Geometry: final body of the model. Coordinates: model frame, mm. Face numbers are marked on the shaded views. Coordinates: 2 decimals unless noted, no trailing zeros. Write each loop counter-clockwise with the first axis right and the second up, starting at its lowest first coordinate (ties: lowest second). Pieces come first, ordered by that corner, then holes.
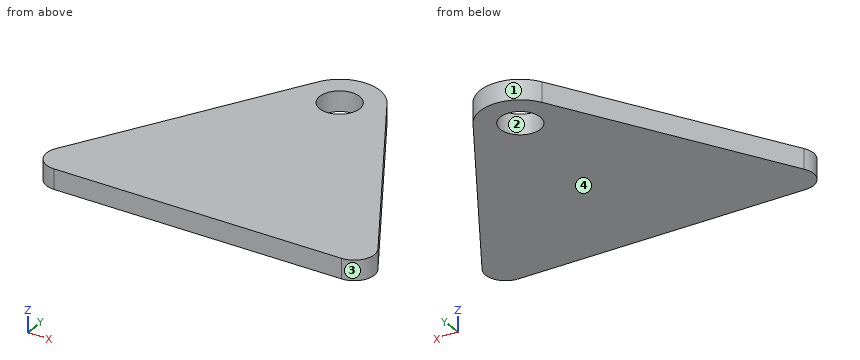
from build123d import *

# Parameters (mm, degrees)
F0_R     = 5
F1_DEPTH = 5


with BuildPart() as f1:
    # F0 (on Top) → F1 (new body)
    with BuildSketch(Plane.XY):
        with BuildLine():
            Line((-35.91768, -56.190782), (0, -56.190782))
            Line((0, -56.190782), (35.91768, -56.190782))
            ThreePointArc((35.91768, -56.190782), (40.258006, -53.673033), (40.227191, -48.65541))
            Line((40.227191, -48.65541), (8.619023, 5.070743))
            ThreePointArc((8.619023, 5.070743), (0, 10), (-8.619023, 5.070743))
            Line((-8.619023, 5.070743), (-40.227191, -48.65541))
            ThreePointArc((-40.227191, -48.65541), (-40.258006, -53.673033), (-35.91768, -56.190782))
        make_face()
        Circle(F0_R, mode=Mode.SUBTRACT)
    extrude(amount=F1_DEPTH)


solid = f1.part
Item 1: Pull-direction query (X, two-part tool) for the marked faces 1, 2, 3 and 4; classes: released by +X, released by -X, zero draft, split by the parting line, or undercut.
Derived:
face 1: split by the parting line
face 2: undercut
face 3: released by +X
face 4: zero draft
Item 2: Section A-A, the plane x = 0. Output: boundary loops of the cut face in (y, z), plus the area to 3 significant figures.
Derived:
outline: (-56.19, 0) - (-5, 0) - (-5, 5) - (-56.19, 5) - close; (5, 0) - (10, 0) - (10, 5) - (5, 5) - close
area: 281 mm2
Item 3: Pin query (flat end, axial travel): pin 1 (1.5 mm diameter, centred on y = -19.5, z = 0.5, fed in from +X); pin 2 (8 mm diameter, centred on x = 0, y = 0, fed in from +Z); pin 3 (2 mm diameter, centred on x = 9.5, z = 1.5, fed in from +Y). Return the tip coordinate at first contact, or that it passes through.
Derived:
pin 1: stops at x = 23.52
pin 2: passes through
pin 3: stops at y = 5.27
Item 4: Section D-D, the plane y = -7.5. Output: boundary loops of the cut face in (x, z).
Derived:
outline: (-16.01, 0) - (16.01, 0) - (16.01, 5) - (-16.01, 5) - close
Item 5: Material intervals for probe 1 along Y at (x, z) = (-10.5, 1.3); probe 2 along Y at (x, z) = (4, 1.45); probe 3 along X at (y, z) = (-2, 1.25), sorted ascending.
Derived:
probe 1: y = -56.19 to 1.87
probe 2: y = -56.19 to -3, 3 to 9.17
probe 3: x = -12.78 to -4.58, 4.58 to 12.78
Item 6: Section B-B, the plane z = 4.2. Output: boundary loops of the cut face in (x, y), plus the area to 3 significant figures.
Derived:
outline: (-40.23, -48.66) arc R5 ccw to (-35.92, -56.19) - (35.92, -56.19) arc R5 ccw to (40.23, -48.66) - (8.62, 5.07) arc R10 ccw to (-8.62, 5.07) - close; hole circle Ø10 at (0, 0)
area: 3,210 mm2
Item 7: Section C-C, the plane y = 0. Output: boundary loops of the cut face in (x, z), plus the area to 3 significant figures.
Derived:
outline: (-11.6, 0) - (-5, 0) - (-5, 5) - (-11.6, 5) - close; (5, 0) - (11.6, 0) - (11.6, 5) - (5, 5) - close
area: 66.0 mm2
